CAD build for the part. Positions are in the model's coordinates, mm. Give positions to 0.01 mm unless a question says otherwise; leave off trailing zeros. Write each loop counter-clockwise with the first axis right and the second up, starting at its lowest first coordinate (ties: lowest second). Pieces come first, ordered by that corner, then holes. Notation, with made-up numbers: M -18.5,57.25 L 15.5,57.25 A20 ccw 15.5,87.25 Z; hole C 65.25,41.5 d8. An arc over 180 degrees is marked long. One line per question, with ' | ' between items. Start each with the question number.
1. Pull direction Z, two halves, no side cores. Call faces 1 (the face through (2.17, 0.99, 9.76)), 2 (the face through (2.614, 0.986, 0.575)), 3 (the face through (0, 2, 0)): released by +Z, released by -Z, zero draft, split by the parting line, or undercut.
2. Wall check: L1, parallel to Z at x = 0, y = 0.7; L2, parallel to Z at x = 4, y = 1.15; L3, parallel to Z at x = -5.25, y = 0.25. Give the ranges that are in metal, low to high.
3. Cut at C-C, the plane y = 1.1. Write the cut outline in (x, z).
4. Cut at D-D, the plane z = -5.25. Write the cut outline in (x, y), then the cut area to 3 significant figures.
5. Cut at A-A, the plane x = 0. Write the cut outline in (y, z), then the cut area to 3 significant figures.
6. Flat gauge pins, fed straight in: pin 1 (1 mm diameter, centred on y = 0.5, z = 6, fed in from -X); pin 2 (8 mm diameter, centred on x = -5, z = -0.5, fed in from +Y); pin 3 (2.5 mm diameter, centred on x = 0, z = 4, fed in from -Y); pin 4 (1 mm diameter, centred on y = 0.5, z = -7, fed in from +X). Where does each tip first touch, or does it go through?
7. Cut at B-B, the plane z = 0. Write the cut outline in (x, y), then the cut area to 3 significant figures.
Autodesk Inventor part; units mm, degrees
ref_plane "YZ Plane" through (0, 0, 0) normal (1, 0, 0) x (0, 1, 0)
ref_plane "XZ Plane" through (0, 0, 0) normal (0, 1, 0) x (-1, 0, 0)
ref_plane "XY Plane" through (0, 0, 0) normal (0, 0, 1) x (1, 0, 0)
sketch "Sketch1" plane through (0, 0, 0) normal (0, 1, 0) x (-1, 0, 0)
  circle A0 centre (0, 0) radius 10
  circle A1 centre (4, 0) radius 1.5
  circle A2 centre (0, 4) radius 1.5
  circle A3 centre (-4, 0) radius 1.5
  circle A4 centre (0, -4) radius 1.5
  dimension "d0" = 20
  dimension "d2" = 3
  dimension "d5" = 360
extrude "Extrusion1" add sketch "Sketch1" along normal blind 2
properties part number "spacer"
Here are the results:
1) face 1: split by the parting line | face 2: undercut | face 3: zero draft
2) L1: -10 to -5.5, -2.5 to 2.5, 5.5 to 10 | L2: -9.17 to -1.5, 1.5 to 9.17 | L3: -8.51 to -0.83, 0.83 to 8.51
3) outline: C 0,0 d20; hole C -4,0 d3; hole C 0,-4 d3; hole C 0,4 d3; hole C 4,0 d3
4) outline: M -8.51,0 L -0.83,0 L -0.83,2 L -8.51,2 Z; M 0.83,0 L 8.51,0 L 8.51,2 L 0.83,2 Z | area: 30.7 mm^2
5) outline: M 0,-10 L 2,-10 L 2,-5.5 L 0,-5.5 Z; M 0,-2.5 L 2,-2.5 L 2,2.5 L 0,2.5 Z; M 0,5.5 L 2,5.5 L 2,10 L 0,10 Z | area: 28.0 mm^2
6) pin 1: x = -8.35 | pin 2: y = 2 | pin 3: through | pin 4: x = 7.6
7) outline: M -10,0 L -5.5,0 L -5.5,2 L -10,2 Z; M -2.5,0 L 2.5,0 L 2.5,2 L -2.5,2 Z; M 5.5,0 L 10,0 L 10,2 L 5.5,2 Z | area: 28.0 mm^2
